Geometry: final body of the model. Coordinates: model frame, mm. A direction names the side the tool comes from. Give positions to 0.01 mm unless a question says otherwise; leave off trailing zeros. Write each loop counter-clockwise with the first axis right and the second up, starting at its lowest first coordinate (ties: lowest second). Pieces come first, ordered by that corner, then holes. Notation, with made-up numbers: (0, 59.5) - (57, 59.5) arc R17 ccw to (57, 81.5) - close; hole circle Ø6 at (20, 40). An arc over 180 degrees is marked (long way). Use CSV: the item, a comma, the result in double quotes. Start each with the question number.
(1) Section C-C on z = -18.5. Output: boundary loops of the cut face in (x, y) (3 decimals), and give its area (3 significant figures).
(2) First-contact query: pin 1 Ø4 at (x, z) = (11, 7.5) entering from -Y; pin 2 Ø6 at (y, z) = (-103, 9.5) entering from -X; pin 3 Ø6 at (y, z) = (-4.5, 10) entering from -X. Flat tips, straight axial feed; report the tip coordinate or a pass-through.
(3) Line query: probe 1 along Y at (x, z) = (43, 19.5); probe 2 along Y at (x, z) = (18, -20); probe 3 along X at (y, z) = (-155.5, -10.5). Output: solid intervals per line, ascending. Write a range as [from, to].
(4) Section D-D on x = -50.5. Output: boundary loops of the cut face in (y, z).
(5) Draft query along X for faces 1 (the flat face through (50.152, -51.266, -0.35)), 2 (the flat face through (-66.664, -51.482, 0.35)), 3 (the flat face through (0, -78, -25)). Return one class per face: released by +X, released by -X, zero draft, split by the parting line, or undercut.
(6) Section A-A on y = -160. Output: boundary loops of the cut face in (x, z), and give its area (3 significant figures).
(7) Section B-B on x = 0. Output: boundary loops of the cut face in (y, z), and give its area (3 significant figures).
(8) Reachability of faces 4 (the cylindrical face through (-0.645, 39.995, 0.35)), 5 (the cylindrical face through (35.085, -27.692, -0.35)) from +Z, -Z, +X, -X, +Y, -Y: full face, straight path, thin tool, end or side. Return the list, or none.
from build123d import *

# Parameters (mm, degrees)
SKETCH1_R               = 75
BOSS_EXTRUDE1_DEPTH     = 25
CUT_EXTRUDE1_DEPTH      = 287.138078556
CUT_EXTRUDE1_DEPTH_BACK = 287.138078556
FILLET1_START           = -25
FILLET1_DEPTH           = 50
SKETCH3_R               = 30
CUT_EXTRUDE2_DEPTH      = 290.39592257


with BuildPart() as part:
    # Sketch1 → Boss-Extrude1 (new, symmetric)
    with BuildSketch(Plane.XY):
        with BuildLine():
            Line((-95.945006832, -117.34375), (-36.550478793, 16.25))
            ThreePointArc((-36.550478793, 16.25), (0, 40), (36.550478793, 16.25))
            Line((36.550478793, 16.25), (95.945006832, -117.34375))
            ThreePointArc((95.945006832, -117.34375), (0, -265), (-95.945006832, -117.34375))
        make_face()
        with Locations((0, -160)):
            Circle(SKETCH1_R, mode=Mode.SUBTRACT)
    extrude(amount=BOSS_EXTRUDE1_DEPTH, both=True)

    # Sketch2 → Cut-Extrude1 (cut, two sides: drawn at the far end of the back side and taken through both)
    with BuildSketch(Plane.XY.offset(-CUT_EXTRUDE1_DEPTH_BACK)):
        with BuildLine():
            Line((-35.52920143, -18.375958363), (-82.238577284, -123.4375))
            ThreePointArc((-82.238577284, -123.4375), (0, -70), (82.238577284, -123.4375))
            Line((82.238577284, -123.4375), (35.52920143, -18.375958363))
            ThreePointArc((35.52920143, -18.375958363), (0, -40), (-35.52920143, -18.375958363))
        make_face()
    extrude(amount=CUT_EXTRUDE1_DEPTH + CUT_EXTRUDE1_DEPTH_BACK, mode=Mode.SUBTRACT)

    # Fillet1: read off the stored shape, not the designer's step
    # Fillet1 outline → Fillet1 (add)
    with BuildSketch(Plane.XY.offset(FILLET1_START)):
        with BuildLine():
            ThreePointArc((-42.220939274, -33.427418189), (-35.213916082, -27.719526256), (-26.466655661, -29.991934551))
            ThreePointArc((-26.466655661, -29.991934551), (-31.537347698, -24.604790188), (-35.52920143, -18.375958363))
            Line((-35.52920143, -18.375958363), (-42.220939274, -33.427418189))
        make_face()
        with BuildLine():
            ThreePointArc((35.52920143, -18.375958363), (31.537347698, -24.604790188), (26.466655661, -29.991934551))
            ThreePointArc((26.466655661, -29.991934551), (35.213916082, -27.719526256), (42.220939274, -33.427418189))
            Line((42.220939274, -33.427418189), (35.52920143, -18.375958363))
        make_face()
        with BuildLine():
            ThreePointArc((-43.853361827, -81.406853629), (-55.469552548, -80.058313703), (-57.863577284, -68.61178181))
            Line((-57.863577284, -68.61178181), (-82.238577284, -123.4375))
            ThreePointArc((-82.238577284, -123.4375), (-66.45628703, -99.30764534), (-43.853361827, -81.406853629))
        make_face()
        with BuildLine():
            Line((82.238577284, -123.4375), (57.863577284, -68.61178181))
            ThreePointArc((57.863577284, -68.61178181), (55.469552548, -80.058313703), (43.853361827, -81.406853629))
            ThreePointArc((43.853361827, -81.406853629), (66.45628703, -99.30764534), (82.238577284, -123.4375))
        make_face()
    extrude(amount=FILLET1_DEPTH)

    # Sketch3 → Cut-Extrude2 (cut, through all)
    with BuildSketch(Plane.XY.offset(25)):
        Circle(SKETCH3_R)
    extrude(amount=-CUT_EXTRUDE2_DEPTH, mode=Mode.SUBTRACT)


solid = part.part
Check values:
1,outline,"(-95.945, -117.344) arc R105 ccw (long way) to (95.945, -117.344) - (36.55, 16.25) arc R40 ccw to (-36.55, 16.25) - close; hole circle Ø150 at (0, -160); hole (-57.864, -68.612) arc R10 ccw to (-43.853, -81.407) arc R90 cw to (43.853, -81.407) arc R10 ccw to (57.864, -68.612) - (42.221, -33.427) arc R10 ccw to (26.467, -29.992) arc R40 cw to (-26.467, -29.992) arc R10 ccw to (-42.221, -33.427) - close; hole circle Ø60 at (0, 0)"
1,area,"20,200 mm²"
2,pin 1,"stops at y = -264.61"
2,pin 2,"stops at x = -90.9"
2,pin 3,"stops at x = -47.11"
3,probe 1,"y = [-255.79, -221.45], [-98.55, -80.94], [-35.18, 1.74]"
3,probe 2,"y = [-263.45, -232.81], [-87.19, -71.82], [-35.72, -24], [24, 35.72]"
3,probe 3,"x = [-104.9, -74.86], [74.86, 104.9]"
4,outline,"(-252.06, -25) - (-215.45, -25) - (-215.45, 25) - (-252.06, 25) - close; (-104.55, -25) - (-82.52, -25) - (-82.52, 25) - (-104.55, 25) - close; (-52.05, -25) - (-15.13, -25) - (-15.13, 25) - (-52.05, 25) - close"
5,face 1,"undercut"
5,face 2,"released by -X"
5,face 3,"zero draft"
6,outline,"(-105, -25) - (-75, -25) - (-75, 25) - (-105, 25) - close; (75, -25) - (105, -25) - (105, 25) - (75, 25) - close"
6,area,"3,000 mm²"
7,outline,"(-265, -25) - (-235, -25) - (-235, 25) - (-265, 25) - close; (-85, -25) - (-70, -25) - (-70, 25) - (-85, 25) - close; (-40, -25) - (-30, -25) - (-30, 25) - (-40, 25) - close; (30, -25) - (40, -25) - (40, 25) - (30, 25) - close"
7,area,"3,250 mm²"
8,face 4,"+Z, -Z, +Y"
8,face 5,"+Z, -Z"
